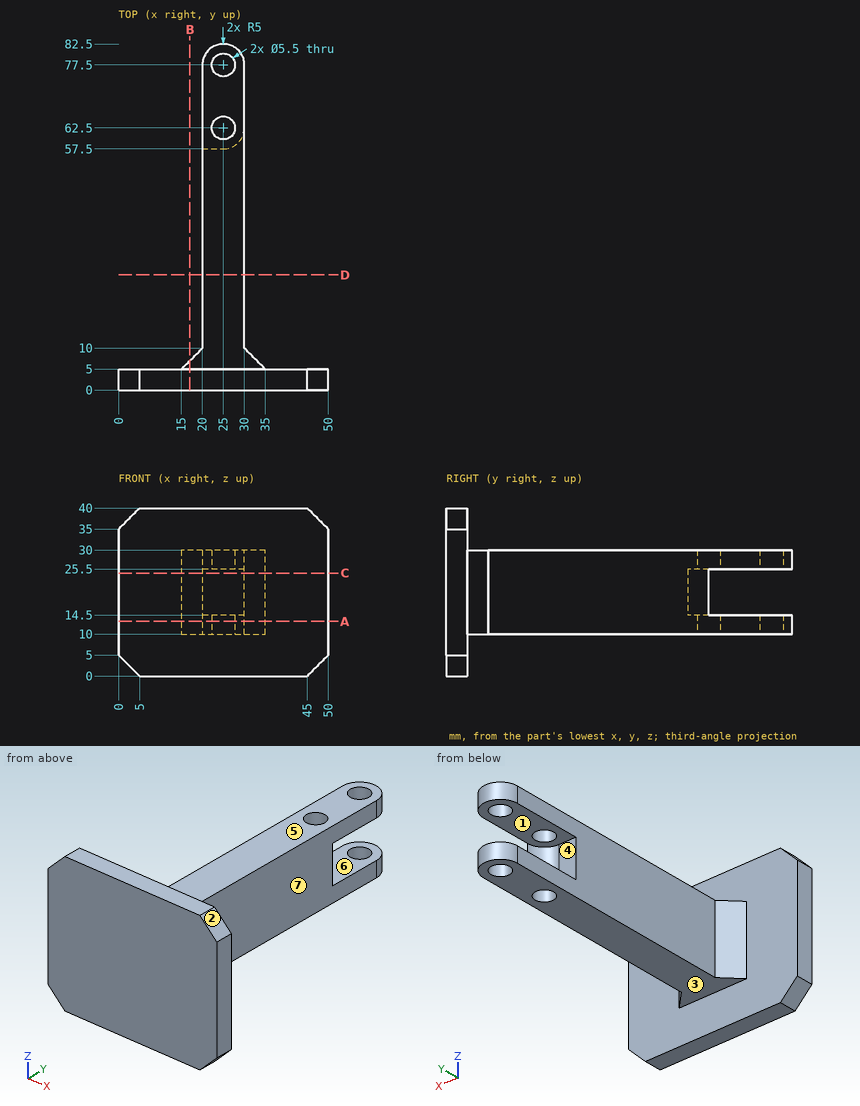
For this review, use the dimensioned drawing (mm, ordinates from the lowest corner) and the shaded views. A direction names the side the tool comes from. Round coordinates to 2 decimals unless told otherwise and drop trailing zeros. Write each loop counter-clockwise with the first axis right and the second up, starting at its lowest first coordinate (ties: lowest second). Pieces come first, ordered by that corner, then holes. Notation, with made-up numbers: (38, -6) - (70, -6) arc R17 cw to (70, 6) - close; hole circle Ø2 at (3, -22.75). An arc over 180 degrees is marked (long way). Answer as a JSON object with one key per item and string values.
1. We need section C-C on z = 24.5. Give the boundary of the cut face in (x, y).
Response values:
{"outline": "(0, 0) - (50, 0) - (50, 5) - (35, 5) - (30, 10) - (30, 62.5) arc R5 cw to (25, 57.5) - (20, 57.5) - (20, 10) - (15, 5) - (0, 5) - close"}
2. We need section B-B on x = 17. Give the boundary of the cut face in (y, z), then the cut area to 3 significant figures.
Response values:
{"outline": "(0, 0) - (5, 0) - (5, 10) - (7, 10) - (7, 30) - (5, 30) - (5, 40) - (0, 40) - close", "area": "240 mm2"}
3. Draft analysis for pull direction Z (two halves, no side actions). For the marked faces 1, 2, 3 and 4, state which applies: +Z half, -Z half, draft (parallel to the pull), parting line (faces both ways), or undercut.
Response values:
{"face 1": "undercut", "face 2": "+Z half", "face 3": "-Z half", "face 4": "undercut"}
4. Tool access review of the marked faces 5, 6 and 7: name each direction out of +Z, -Z, +X, -X, +Y, -Y from which nothing blocks a thin tool from reaching the whole face with its end or side.
Response values:
{"face 5": "+Z, +X, -X, +Y", "face 6": "-X, +Y", "face 7": "+Z, -Z, +X, +Y"}
5. To check wall thickness, follow line 1 along Y through (x, z) = (25, 28); line 2 along Y through (x, z) = (18.5, 37); line 3 along X through (y, z) = (19, 29). State the ranges of each line that lie inside material, in increasing order.
Response values:
{"line 1": "y = 0 to 59.75, 65.25 to 74.75, 80.25 to 82.5", "line 2": "y = 0 to 5", "line 3": "x = 20 to 30"}
6. For pin 1 Ø22 at (y, z) = (56.5, 24) entering from +X; pin 2 Ø5 at (x, y) = (23.5, 71) entering from -Z; pin 3 Ø10 at (x, z) = (33, 9.5) entering from +Y, all flat-tipped, find the tip position at first contact; note any pin that passes through.
Response values:
{"pin 1": "stops at x = 30", "pin 2": "stops at z = 10", "pin 3": "stops at y = 81.48"}
7. We need section D-D on y = 27.5. Give the boundary of the cut face in (x, z), then the cut area to 3 significant figures.
Response values:
{"outline": "(20, 10) - (30, 10) - (30, 30) - (20, 30) - close", "area": "200 mm2"}
8. We need section A-A on z = 13. Give the boundary of the cut face in (x, y).
Response values:
{"outline": "(0, 0) - (50, 0) - (50, 5) - (35, 5) - (30, 10) - (30, 77.5) arc R5 ccw to (20, 77.5) - (20, 10) - (15, 5) - (0, 5) - close; hole circle Ø5.5 at (25, 62.5); hole circle Ø5.5 at (25, 77.5)"}
